Could you check a few things on this model? Use its own coordinates, in mm. A direction names the side the tool comes from. Coordinates: 2 decimals unless noted, no trailing zeros. Write each loop counter-clockwise with the first axis right and the second up, starting at its lowest first coordinate (ties: lowest second). Pieces come first, ordered by that corner, then holes.
```python
from build123d import *

# Parameters (mm, degrees)
F1_ANGLE_BACK = 30
F1_ANGLE      = 75
F2_R          = 3
F3_R          = 3


with BuildPart() as f1:
    # F0 (on Top) → F1 (revolve)
    with BuildSketch(Plane.XY, mode=Mode.PRIVATE) as f1_sk:
        with BuildLine():
            ThreePointArc((24.5736017823, 111.5037277341), (0.2955596523, 87.4353562361), (-8.600258129, 54.4266564399))
            Line((-8.600258129, 54.4266564399), (-8.600258129, 24.4266564399))
            Line((-8.600258129, 24.4266564399), (8.399741871, 24.4266564399))
            Line((8.399741871, 24.4266564399), (8.399741871, 27.4266564399))
            Line((8.399741871, 27.4266564399), (-1.600258129, 27.4266564399))
            Line((-1.600258129, 27.4266564399), (-1.600258129, 54.4266564399))
            ThreePointArc((-1.600258129, 54.4266564399), (4.1886480826, 83.1872765912), (20.6537842751, 107.4686273932))
            Line((20.6537842751, 107.4686273932), (21.2201206089, 108.0516198232))
            ThreePointArc((21.2201206089, 108.0516198232), (21.6429306698, 109.0350473427), (22.6136930287, 109.4861775637))
            Line((22.6136930287, 109.4861775637), (24.5736017823, 111.5037277341))
        make_face()
    revolve(f1_sk.sketch.rotate(Axis((5.6419791654, -475.5733435601, 0), (1, 0, 0)), -F1_ANGLE_BACK), axis=Axis((5.6419791654, -475.5733435601, 0), (1, 0, 0)), revolution_arc=F1_ANGLE)

    # F2
    f2_edges = [f1.edges().sort_by_distance(p)[0] for p in [
        (-8.600258, 20.149087, 65.263096),
    ]]
    fillet(f2_edges, radius=F2_R)

    # F3
    f3_edges = [f1.edges().sort_by_distance(p)[0] for p in [
        (-1.600258, 23.123422, 65.654675),
    ]]
    fillet(f3_edges, radius=F3_R)


solid = f1.part
```
1. For pin 1 (1 mm diameter, centred on x = 1.5, z = 284.5, fed in from -Y); pin 2 (1 mm diameter, centred on x = 19, z = 213.5, fed in from +Y); pin 3 (5 mm diameter, centred on y = -12, z = 271, fed in from -X), each with a flat end and sliding along its axis, tell me the tip position at first contact or that it passes through.
Verdict:
pin 1: stops at y = -64.75
pin 2: stops at y = 67.91
pin 3: stops at x = -8.45
2. On a 3-axis mill with a long thin cutter (end or side, diameter ignored), from which of +Z, -Z, +X, -X, +Y, -Y can I reach the whole of each face in a straight line? I mean faces 1 (the face through (1.498, 20.726, 60.718)), 2 (the face through (4.9, 23.7, 61.1)). Say none if no direction works.
Verdict:
face 1: +X, -X, -Y
face 2: +X
3. Please list where these lines run through material, in increasing order: line 1 along X through (y, z) = (-100, 343.5); line 2 along Y through (x, z) = (10.5, 60); line 3 along Y through (x, z) = (21, -147).
Verdict:
line 1: x = -8.6 to -1.6
line 2: y = 91.92 to 97.6
line 3: y = 89 to 90.54
4. If we mould it in two halves opening along Z, with no side actions, what happens to faces 3 (the face through (-1.6, 32, 69)), 4 (the face through (-1.92, -97.931, 377.642)), 5 (the face through (-1.92, -13.06, -267.03))? For each: pulls with the +Z half, pulls with the -Z half, needs draft (parallel to the pull), parting line crosses it, or undercut.
Verdict:
face 3: undercut
face 4: pulls with the +Z half
face 5: pulls with the -Z half
5. I want a section at A-A on x = 15.5. Please give me the cut outline in (y, z).
Verdict:
outline: (-67.27, 408.31) arc R577.43 cw to (24.5, -288.72) - (27.45, -290.42) arc R580.85 ccw to (-64.85, 410.72) - close
